Source: CAD feature listing. Evaluate the final solid. Frame: model axes, mm. Face numbers are marked on the shaded views. A direction names the side the tool comes from. Give positions to 0.01 mm unless a question says otherwise; leave off trailing zeros. Write each loop counter-clockwise with the first axis right and the second up, starting at its lowest first coordinate (ties: lowest second). Pieces come first, ordered by that corner, then holes. Notation, with made-up numbers: (67.5, 84.25) - (117.5, 84.25) arc R23 ccw to (117.5, 105.25) - close; hole circle Ø4 at (29.5, 25). An arc over 180 degrees is marked (long way). Answer as a JSON object with one key per item and string values. Group by question number.
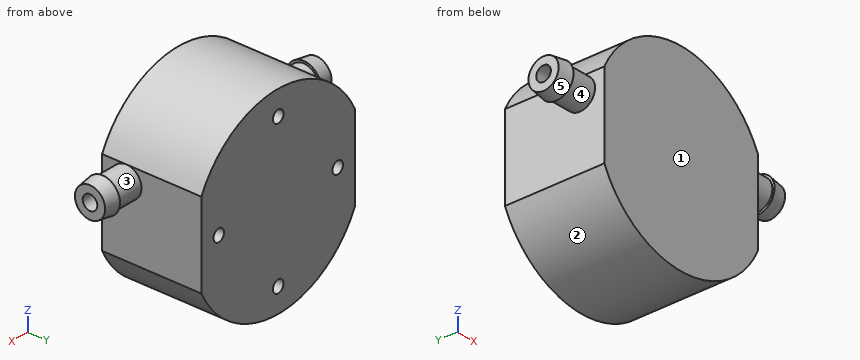
from build123d import *

# Parameters (mm, degrees)
BOSS_EXTRUDE1_DEPTH       = 20.4
M3X0_5_TAPPED_HOLE1_D     = 2.5
M3X0_5_TAPPED_HOLE1_DEPTH = 7.5
M3X0_5_TAPPED_HOLE1_TIP   = 0.751075774
BOSS_EXTRUDE3_DEPTH       = 8.6
BOSS_EXTRUDE3_DEPTH_BACK  = 44.9
SKETCH5_R                 = 3.1
SKETCH8_R                 = 1.5
CUT_EXTRUDE1_DEPTH        = 61.682946534


with BuildPart() as part:
    # Sketch1 → Boss-Extrude1 (new body)
    with BuildSketch(Plane(origin=(0, 0, 0), x_dir=(1, 0, 0), z_dir=(0, 1, 0))):
        with BuildLine():
            Line((-18.15, -8.636405502), (-18.15, 8.636405502))
            ThreePointArc((-18.15, 8.636405502), (0, 20.1), (18.15, 8.636405502))
            Line((18.15, 8.636405502), (18.15, -8.636405502))
            ThreePointArc((18.15, -8.636405502), (0, -20.1), (-18.15, -8.636405502))
        make_face()
    extrude(amount=-BOSS_EXTRUDE1_DEPTH)

    # M3x0.5 Tapped Hole1
    with Locations(Plane(origin=(0, 0, 0), x_dir=(1, 0, 0), z_dir=(0, 1, 0))):
        with Locations((0, 15.15), (0, -15.15), (14.05, 0), (-14.05, 0)):
            Hole(M3X0_5_TAPPED_HOLE1_D / 2, depth=M3X0_5_TAPPED_HOLE1_DEPTH)
            with Locations((0, 0, -(M3X0_5_TAPPED_HOLE1_DEPTH + M3X0_5_TAPPED_HOLE1_TIP / 2))):  # 118° drill point
                Cone(0, M3X0_5_TAPPED_HOLE1_D / 2, M3X0_5_TAPPED_HOLE1_TIP, mode=Mode.SUBTRACT)

    # Sketch5 → Boss-Extrude3 (add, two sides: drawn at the far end of the back side and taken through both)
    with BuildSketch(Plane(origin=(18.15, 0, 0), x_dir=(0, 0, -1), z_dir=(1, 0, 0)).offset(-BOSS_EXTRUDE3_DEPTH_BACK)):
        with Locations(Location((-5.536405502, -15.4, 0), (0, 0, 180))):
            Circle(SKETCH5_R)
    extrude(amount=BOSS_EXTRUDE3_DEPTH + BOSS_EXTRUDE3_DEPTH_BACK)

    # Sketch7 → Revolve1 (revolve)
    with BuildSketch(Plane.XY.offset(5.536405502), mode=Mode.PRIVATE) as revolve1_sk:
        Polygon((26.75, -12.3), (23.75, -11.85), (23.75, -12.3), align=None)
        Polygon((-26.75, -12.3), (-23.75, -11.85), (-23.75, -12.3), align=None)
    revolve(revolve1_sk.sketch.rotate(Axis((26.75, -15.4, 5.536405502), (-1, 0, 0)), 270), axis=Axis((26.75, -15.4, 5.536405502), (-1, 0, 0)))

    # Sketch8 → Cut-Extrude1 (cut, through all)
    with BuildSketch(Plane(origin=(26.75, 0, 0), x_dir=(0, 0, -1), z_dir=(1, 0, 0))):
        with Locations((-5.536405502, -15.4)):
            Circle(SKETCH8_R)
    extrude(amount=-CUT_EXTRUDE1_DEPTH, mode=Mode.SUBTRACT)


solid = part.part
Q1. Ray query, probe 1 along Y at (x, z) = (9.5, 5.5); probe 2 along X at (y, z) = (-10.5, 4); probe 3 along Z at (x, y) = (14.5, -5). Return the intervals inside material, ascending. Write a range as [from, to].
Q2. Section D-D on x = -12. Return the cut outline in (y, z), then the cut area to 3 significant figures.
Q3. Reachability of the marked faces 4 and 5 from +Z, -Z, +X, -X, +Y, -Y: full face, straight path, thin tool, end or side. Return the list, or none.
Q4. Section C-C on z = 17. Return the cut outline in (x, y).
Q5. Section A-A on x = -21. Return the cut outline in (y, z).
Q6. Section B-B on y = -11.25. Return the cut outline in (x, z), then the cut area to 3 significant figures.
Q7. Draft query along X for the marked faces 1, 2 and 3. Return one class per face: released by +X, released by -X, zero draft, split by the parting line, or undercut.
Q8. First-contact query: pin 1 Ø6 at (x, y) = (4, -4) entering from -Z; pin 2 Ø1.5 at (x, z) = (0, 15.15) entering from +Y; pin 3 Ø2 at (x, z) = (0, -15.15) entering from +Y. Flat tips, straight axial feed; report the tip coordinate or a pass-through.
Taken from the geometry:
{
 "1": {"probe 1": "y = [-20.4, -16.9], [-13.9, 0]", "probe 2": "x = [-18.15, 18.15]", "probe 3": "z = [-13.92, -1.17], [1.17, 13.92]"},
 "2": {"outline": "(-20.4, -16.12) - (0, -16.12) - (0, 16.12) - (-20.4, 16.12) - close; hole circle Ø3 at (-15.4, 5.54)", "area": "651 mm²"},
 "3": {"face 4": "none", "face 5": "-X"},
 "4": {"outline": "(-10.72, -20.4) - (10.72, -20.4) - (10.72, 0) - (-10.72, 0) - close"},
 "5": {"outline": "circle Ø6.2 at (-15.4, 5.54); hole circle Ø3 at (-15.4, 5.54)"},
 "6": {"outline": "(-18.15, -8.64) arc R20.1 ccw to (18.15, -8.64) - (18.15, 8.64) arc R20.1 ccw to (-18.15, 8.64) - close", "area": "1,220 mm²"},
 "7": {"face 1": "zero draft", "face 2": "split by the parting line", "face 3": "undercut"},
 "8": {"pin 1": "stops at z = -20.08", "pin 2": "stops at y = -7.8", "pin 3": "stops at y = -7.65"}
}
